The figure shows three views and two pictorial views of one solid part (mm, origin at its lowest corner). Answer the questions. A direction names the side the tool comes from. Coordinates: 2 decimals unless noted, no trailing zeros. Order: outer loops, then holes, each group sorted by start corner. A loop starts at its lowest first (then second) coordinate and runs counter-clockwise, first axis right, second up.
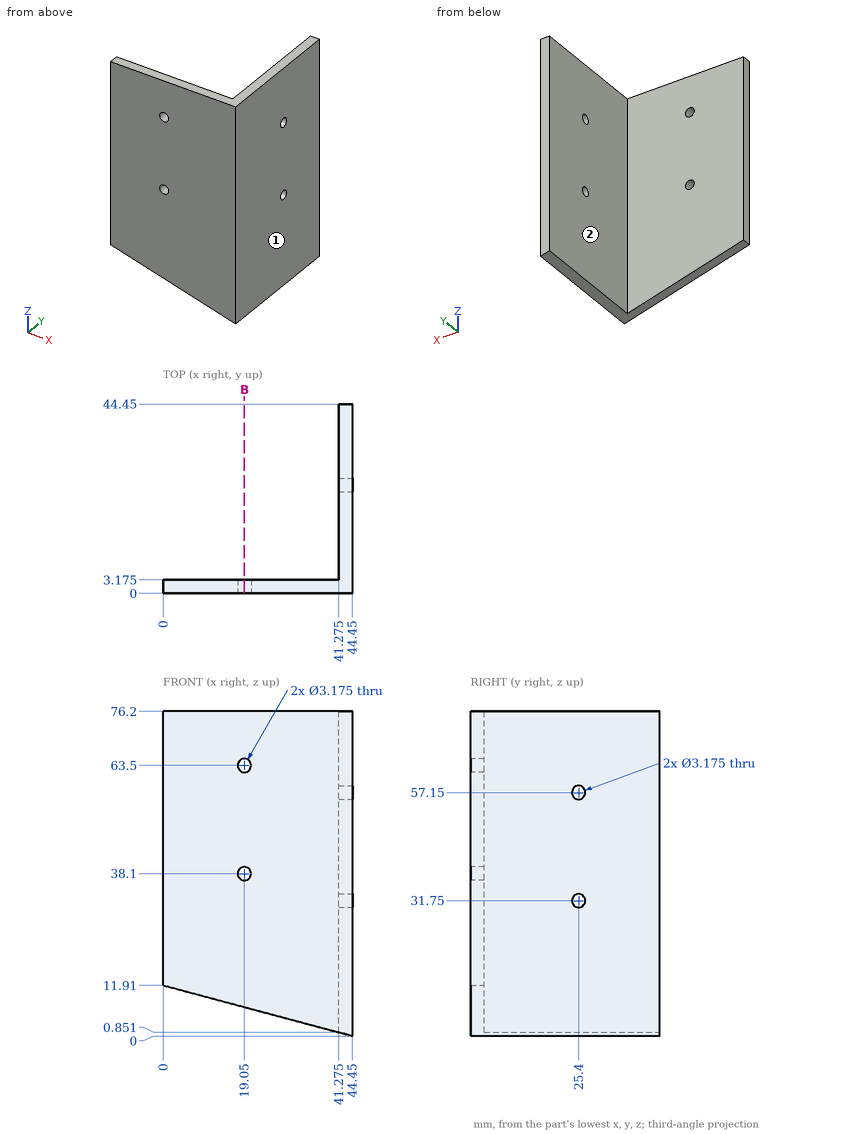
1) Each of these flat-tipped pins is pushed along its axis until it touches: P1, Ø2.5, axis at x = 19.05, z = 63.5, coming from the -Y side; P2, Ø12.5, axis at y = 28, z = 20.5, coming from the -X side (3 decimals). Where does it stop, or does it pass through?
2) A cutting plane is placed at B-B, the plane x = 19.05. Write down the section's boundary in (y, z) (1 decimal), plus the area to 3 significant figures.
3) Straight lines are drawn through the part: probe 1 along X at (y, z) = (2.3, 38.1); probe 2 along Y at (x, z) = (43.25, 31.75); probe 3 along Z at (x, y) = (19, 2). For each, find the intervals that lie inside material, in ascending order.
4) For the marked faces 1 and 2, determine the directions among +Z, -Z, +X, -X, +Y, -Y from which every point of the face is accessible in a straight line to the end or side of a thin tool.
Working result:
1. P1: passes through
1. P2: stops at x = 41.275
2. outline: (0, 6.8) - (3.2, 6.8) - (3.2, 36.5) - (0, 36.5) - close; (0, 39.7) - (3.2, 39.7) - (3.2, 61.9) - (0, 61.9) - close; (0, 65.1) - (3.2, 65.1) - (3.2, 76.2) - (0, 76.2) - close
2. area: 200 mm2
3. probe 1: x = 0 to 17.46, 20.64 to 44.45
3. probe 2: y = 0 to 23.81, 26.99 to 44.45
3. probe 3: z = 6.82 to 36.51, 39.69 to 61.91, 65.09 to 76.2
4. face 1: +Z, -Z, +X, +Y, -Y
4. face 2: +Z, -Z, -X, +Y
